```python
from build123d import *

# Parameters (mm, degrees)
ESQUISSE1_R        = 3
ESQUISSE1_W        = 40
ESQUISSE1_H        = 80
BOSS_EXTRU_1_DEPTH = 5


with BuildPart() as part:
    # Esquisse1 → Boss.-Extru.1 (new body)
    # profile 1 of 7: a face of its own
    with BuildSketch(Plane(origin=(0, 0, 0), x_dir=(1, 0, 0), z_dir=(0, 1, 0))):
        with BuildLine():
            Line((-144.568322948, 130), (-144.568322948, 40))
            ThreePointArc((-144.568322948, 40), (-90.829510466, 119.373363982), (3.94e-07, 150))
            Line((3.94e-07, 150), (-124.568322948, 150))
            Line((-124.568322948, 150), (-124.568322948, 130))
            Line((-124.568322948, 130), (-144.568322948, 130))
        make_face()
    # profile 2 of 7: a face of its own
    with BuildSketch(Plane(origin=(0, 0, 0), x_dir=(1, 0, 0), z_dir=(0, 1, 0))):
        with BuildLine():
            ThreePointArc((3.94e-07, 150), (-90.829510466, 119.373363982), (-144.568322948, 40))
            Line((-144.568322948, 40), (-104.568322948, 40))
            Line((-104.568322948, 40), (-104.568322948, -40))
            Line((-104.568322948, -40), (-144.568322948, -40))
            ThreePointArc((-144.568322948, -40), (-90.829510457, -119.373363989), (4.17e-07, -150))
            ThreePointArc((4.17e-07, -150), (90.829510789, -119.373363737), (144.568322948, -40))
            Line((144.568322948, -40), (104.568322948, -40))
            Line((104.568322948, -40), (104.568322948, 40))
            Line((104.568322948, 40), (144.568322948, 40))
            ThreePointArc((144.568322948, 40), (90.82951078, 119.373363744), (3.94e-07, 150))
        make_face()
        with Locations(Location((-60, -124.57, 0), (0, 0, 270))):
            Circle(ESQUISSE1_R, mode=Mode.SUBTRACT)
        with Locations(Location((60, -124.57, 0), (0, 0, 270))):
            Circle(ESQUISSE1_R, mode=Mode.SUBTRACT)
        with Locations(Location((-60, 124.57, 0), (0, 0, 270))):
            Circle(ESQUISSE1_R, mode=Mode.SUBTRACT)
        with Locations(Location((60, 124.57, 0), (0, 0, 270))):
            Circle(ESQUISSE1_R, mode=Mode.SUBTRACT)
    # profile 3 of 7: a face of its own
    with BuildSketch(Plane(origin=(0, 0, 0), x_dir=(1, 0, 0), z_dir=(0, 1, 0))):
        with BuildLine():
            ThreePointArc((4.17e-07, -150), (-90.829510457, -119.373363989), (-144.568322948, -40))
            Line((-144.568322948, -40), (-144.568322948, -130))
            Line((-144.568322948, -130), (-124.568322948, -130))
            Line((-124.568322948, -130), (-124.568322948, -150))
            Line((-124.568322948, -150), (4.17e-07, -150))
        make_face()
    # profile 4 of 7: a face of its own
    with BuildSketch(Plane(origin=(0, 0, 0), x_dir=(1, 0, 0), z_dir=(0, 1, 0))):
        with BuildLine():
            ThreePointArc((144.568322948, -40), (90.829510789, -119.373363737), (4.17e-07, -150))
            Line((4.17e-07, -150), (124.568322948, -150))
            Line((124.568322948, -150), (124.568322948, -130))
            Line((124.568322948, -130), (144.568322948, -130))
            Line((144.568322948, -130), (144.568322948, -40))
        make_face()
    # profile 5 of 7: a face of its own
    with BuildSketch(Plane(origin=(0, 0, 0), x_dir=(1, 0, 0), z_dir=(0, 1, 0))):
        with BuildLine():
            Line((124.568322948, 150), (3.94e-07, 150))
            ThreePointArc((3.94e-07, 150), (90.82951078, 119.373363744), (144.568322948, 40))
            Line((144.568322948, 40), (144.568322948, 130))
            Line((144.568322948, 130), (124.568322948, 130))
            Line((124.568322948, 130), (124.568322948, 150))
        make_face()
    # profile 6 of 7: a face of its own
    with BuildSketch(Plane(origin=(0, 0, 0), x_dir=(1, 0, 0), z_dir=(0, 1, 0))):
        with Locations((-124.568322948, 0)):
            Rectangle(ESQUISSE1_W, ESQUISSE1_H)
    # profile 7 of 7: a face of its own
    with BuildSketch(Plane(origin=(0, 0, 0), x_dir=(1, 0, 0), z_dir=(0, 1, 0))):
        with Locations((124.568322948, 0)):
            Rectangle(ESQUISSE1_W, ESQUISSE1_H)
    extrude(amount=BOSS_EXTRU_1_DEPTH)


solid = part.part
```
CAD build for the part. Positions are in the model's coordinates, mm. Give positions to 0.01 mm unless a question says otherwise; leave off trailing zeros. Order: outer loops, then holes, each group sorted by start corner. A loop starts at its lowest first (then second) coordinate and runs counter-clockwise, first axis right, second up.
(1) Flat gauge pins, fed straight in: pin 1 (2.5 mm diameter, centred on x = 136.5, y = 1.5, fed in from +Z); pin 2 (5 mm diameter, centred on x = -60, z = 124.57, fed in from +Y); pin 3 (2.5 mm diameter, centred on x = -134.5, y = 2.5, fed in from -Z); pin 4 (1.5 mm diameter, centred on y = 1.5, z = 145, fed in from -X). Where does each tip first touch, or does it go through?
(2) Saw through at A-A, the plane y = 2.3. Give the cut face in (x, z).
(3) Drill centre lines: L1, parallel to X at y = 2.2, z = 124.57; L2, parallel to Z at x = 126.5, y = 4.55. Where is each one in solid material? Low to high.
Results found:
1. pin 1: stops at z = 130
1. pin 2: passes through
1. pin 3: stops at z = -130
1. pin 4: stops at x = -124.57
2. outline: (-144.57, -130) - (-124.57, -130) - (-124.57, -150) - (124.57, -150) - (124.57, -130) - (144.57, -130) - (144.57, 130) - (124.57, 130) - (124.57, 150) - (-124.57, 150) - (-124.57, 130) - (-144.57, 130) - close; hole circle Ø6 at (-60, -124.57); hole circle Ø6 at (-60, 124.57); hole circle Ø6 at (60, -124.57); hole circle Ø6 at (60, 124.57)
3. L1: x = -144.57 to -63, -57 to 57, 63 to 144.57
3. L2: z = -130 to 130
